Study the drawing (mm; zero at the part's minimum x, y, z) and answer. A direction names the side the tool comes from. Round coordinates to 2 decimals unless told otherwise and drop trailing zeros. Order: outer loops, then holes, each group sorted by start corner. A loop starts at its lowest first (then second) coordinate and runs counter-clockwise, first axis right, second up. Notation, with made-up numbers: (77, 80.5) - (82, 80.5) arc R34 ccw to (82, 110.5) - close; hole circle Ø7 at (-24.75, 51). An arc over 180 degrees is marked (long way). Put each result on its own line as item: value. Start each with the question number.
Q1. Section B-B on y = 12.7 is taken. Give the vertices of the cut face in (x, z).
Q2. Which of the six approach directions +Z, -Z, +X, -X, +Y, -Y give full straight-line access (tool end or side, diameter ignored) to the marked faces 1 and 2?
Q3. Section D-D on z = 5.08 is taken. Give the vertices of the cut face in (x, y), then the cut area to 3 significant figures.
Q4. Section C-C on z = 28.5 is taken. Give the vertices of the cut face in (x, y).
Q5. Find the intervals of material crossed by line 1 along Z through (x, y) = (23.9, 12.7); line 2 along X through (y, z) = (1.75, 14.5); line 3 along Y through (x, z) = (24.6, 5.08), in increasing order. Write a range as from..to.
Q6. Each of these flat-tipped pins is pushed along its axis until it touches: pin 1 Ø6 at (x, z) = (13, 27) entering from +Y; pin 2 Ø1 at (x, z) = (20, 28.5) entering from +Y; pin 3 Ø6 at (y, z) = (14, 30.5) entering from -X. Where does it stop, or does it pass through?
Q7. Section A-A on x = 8.75 is taken. Give the vertices of the cut face in (y, z).
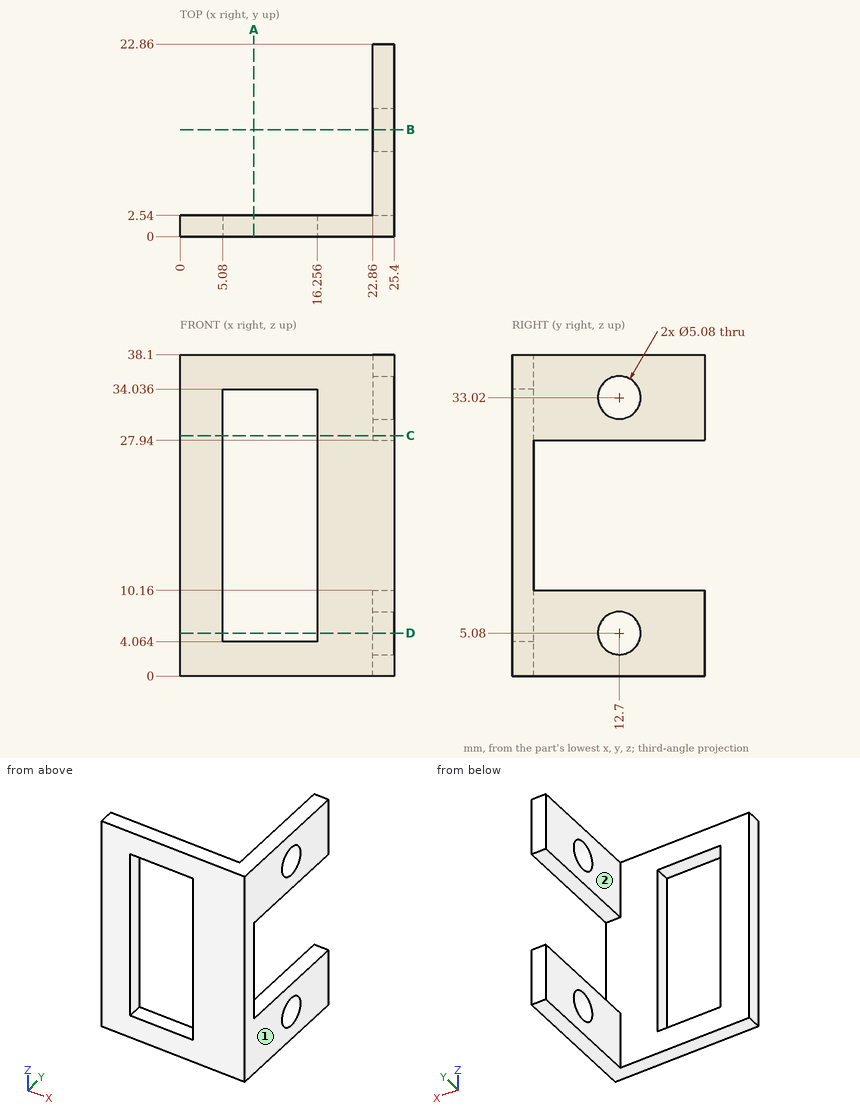
Findings:
1. outline: (22.86, 0) - (25.4, 0) - (25.4, 2.54) - (22.86, 2.54) - close; (22.86, 7.62) - (25.4, 7.62) - (25.4, 10.16) - (22.86, 10.16) - close; (22.86, 27.94) - (25.4, 27.94) - (25.4, 30.48) - (22.86, 30.48) - close; (22.86, 35.56) - (25.4, 35.56) - (25.4, 38.1) - (22.86, 38.1) - close
2. face 1: +Z, -Z, +X, +Y, -Y
2. face 2: +Z, -Z, -X, +Y
3. outline: (0, 0) - (5.08, 0) - (5.08, 2.54) - (0, 2.54) - close; (16.26, 0) - (25.4, 0) - (25.4, 10.16) - (22.86, 10.16) - (22.86, 2.54) - (16.26, 2.54) - close; (22.86, 15.24) - (25.4, 15.24) - (25.4, 22.86) - (22.86, 22.86) - close
3. area: 74.8 mm2
4. outline: (0, 0) - (5.08, 0) - (5.08, 2.54) - (0, 2.54) - close; (16.26, 0) - (25.4, 0) - (25.4, 22.86) - (22.86, 22.86) - (22.86, 2.54) - (16.26, 2.54) - close
5. line 1: 0..2.54, 7.62..10.16, 27.94..30.48, 35.56..38.1
5. line 2: 0..5.08, 16.26..25.4
5. line 3: 0..10.16, 15.24..22.86
6. pin 1: through
6. pin 2: y = 2.54
6. pin 3: x = 22.86
7. outline: (0, 0) - (2.54, 0) - (2.54, 4.06) - (0, 4.06) - close; (0, 34.04) - (2.54, 34.04) - (2.54, 38.1) - (0, 38.1) - close
